from build123d import *

# Parameters (mm, degrees)
F0_W     = 5
F0_H     = 2.0000003874
F1_DEPTH = 10
F2_R     = 4
F3_R     = 3
F4_R     = 1
F5_R     = 1
F6_R     = 1


with BuildPart() as f1:
    # F0 (on Top) → F1 (new body)
    with BuildSketch(Plane.XY):
        with BuildLine():
            ThreePointArc((0, -6), (-6, 0), (0, 6))
            Line((0, 6), (0, 8.9999996126))
            ThreePointArc((0, 8.9999996126), (-8.9999996126, 0), (0, -8.9999996126))
            Line((0, -8.9999996126), (0, -6))
        make_face()
        Polygon((0, 8.9999996126), (0, 6), (3, 6), (3, 14), (0, 14), (0, 11.9999996126), align=None)
        with Locations((-2.5, 12.9999998063)):
            Rectangle(F0_W, F0_H)
        Polygon((3, -6), (0, -6), (0, -8.9999996126), (0, -11.9999996126), (0, -14), (3, -14), align=None)
        with Locations((-2.5, -12.9999998063)):
            Rectangle(F0_W, F0_H)
    extrude(amount=F1_DEPTH)

    # F2
    f2_edges = [f1.edges().sort_by_distance(p)[0] for p in [
        (3, -6, 5),
        (3, 6, 5),
    ]]
    fillet(f2_edges, radius=F2_R)

    # F3
    f3_edges = [f1.edges().sort_by_distance(p)[0] for p in [
        (3, -14, 5),
        (3, 14, 5),
    ]]
    fillet(f3_edges, radius=F3_R)

    # F4
    f4_edges = [f1.edges().sort_by_distance(p)[0] for p in [
        (0, 12, 5),
        (0, -12, 5),
    ]]
    fillet(f4_edges, radius=F4_R)

    # F5
    f5_edges = [f1.edges().sort_by_distance(p)[0] for p in [
        (0, 9, 5),
        (0, -9, 5),
    ]]
    fillet(f5_edges, radius=F5_R)

    # F6
    f6_edges = [f1.edges().sort_by_distance(p)[0] for p in [
        (-5, 12, 5),
        (-5, 14, 5),
        (-5, -12, 5),
        (-5, -14, 5),
    ]]
    fillet(f6_edges, radius=F6_R)


solid = f1.part
Geometry check sheet. Reference: the model listing, model coordinates, mm. A direction names the side the tool comes from. Coordinates: 2 decimals unless noted, no trailing zeros. Order: outer loops, then holes, each group sorted by start corner. A loop starts at its lowest first (then second) coordinate and runs counter-clockwise, first axis right, second up. Notation, with made-up numbers: (47, 26.5) - (95, 26.5) arc R20 cw to (95, 58.5) - close; hole circle Ø11 at (63, 26.5). An arc over 180 degrees is marked (long way). Answer in a Markdown table with one row per item. Add a question column.
1) Cross-section at A-A, the plane x = -2.25. Record the cut outline in (y, z).
2) Set-up check for faces 1 (the cylindrical face through (-0.265, 9.271, 5.07)), 2 (the cylindrical face through (-6, 0, 5)): record each of +Z, -Z, +X, -X, +Y, -Y from which the full face is reachable in a straight line by a thin tool's end or side.
3) Cross-section at C-C, the plane x = -8. Record the cut outline in (y, z).
4) Material ranges on line 1 along Y through (x, z) = (-3.25, 6.25); line 2 along Y through (x, z) = (-0.5, 7.5); line 3 along X through (y, z) = (11, 2.25), recorded low to high. Write a range as [from, to].
5) Cross-section at B-B, the plane y = 4.25. Record the cut outline in (x, z).
6) Release check for a two-part mould opening along Y. For faces 3 (the cylindrical face through (2.14, -13.1, 5.07)), 4 (the flat face through (-6, -3, 10)), 5 (the flat face through (0, -10.5, 4.9)) record: +Y half, -Y half, draft (parallel to the pull), parting line (faces both ways), or undercut.
7) Gauge pin test, flat ends, axial feed: P1, Ø0.5, axis at y = 10.5, z = 7.5, coming from the -X side; P2, Ø3, axis at y = -5.5, z = 2, coming from the +X side; P3, Ø3, axis at y = 7, z = 3.5, coming from the +X side. Record the tip position at first contact, or that the pin passes through.
Check result:
| question | item | result |
|---|---|---|
| 1 | outline | (-14, 0) - (-12, 0) - (-12, 10) - (-14, 10) - close; (-8.71, 0) - (-5.56, 0) - (-5.56, 10) - (-8.71, 10) - close; (5.56, 0) - (8.71, 0) - (8.71, 10) - (5.56, 10) - close; (12, 0) - (14, 0) - (14, 10) - (12, 10) - close |
| 2 | face 1 | +Z, -Z, -X |
| 2 | face 2 | +Z, -Z, +X |
| 3 | outline | (-4.12, 0) - (4.12, 0) - (4.12, 10) - (-4.12, 10) - close |
| 4 | line 1 | y = [-14, -12], [-8.39, -5.04], [5.04, 8.39], [12, 14] |
| 4 | line 2 | y = [-14, -11.87], [-9.08, -5.98], [5.98, 9.08], [11.87, 14] |
| 4 | line 3 | x = [0, 3] |
| 5 | outline | (-7.93, 0) - (-4.24, 0) - (-4.24, 10) - (-7.93, 10) - close |
| 6 | face 3 | -Y half |
| 6 | face 4 | draft |
| 6 | face 5 | undercut |
| 7 | P1 | stops at x = 0 |
| 7 | P2 | stops at x = 1.7 |
| 7 | P3 | stops at x = 2.73 |
